```python
from build123d import *

# Parameters (mm, degrees)
SKETCH1_R           = 4.5
SKETCH1_R_2         = 2
BOSS_EXTRUDE1_DEPTH = 4


with BuildPart() as part:
    # Sketch1 → Boss-Extrude1 (new body)
    with BuildSketch(Plane(origin=(0, 0, 0), x_dir=(1, 0, 0), z_dir=(0, 1, 0))):
        with BuildLine():
            Line((-270, 15), (270, 15))
            ThreePointArc((270, 15), (285, 0), (270, -15))
            Line((270, -15), (-270, -15))
            ThreePointArc((-270, -15), (-285, 0), (-270, 15))
        make_face()
        with Locations(Location((-270, 0, 0), (0, 0, 270))):
            Circle(SKETCH1_R, mode=Mode.SUBTRACT)
        with Locations(Location((270, 0, 0), (0, 0, 270))):
            Circle(SKETCH1_R, mode=Mode.SUBTRACT)
        with Locations(Location((-150, 0, 0), (0, 0, 270))):
            Circle(SKETCH1_R_2, mode=Mode.SUBTRACT)
        with Locations(Location((150, 0, 0), (0, 0, 270))):
            Circle(SKETCH1_R_2, mode=Mode.SUBTRACT)
        with Locations(Location((0, 0, 0), (0, 0, 270))):
            Circle(SKETCH1_R_2, mode=Mode.SUBTRACT)
        with Locations(Location((-250, 0, 0), (0, 0, 270))):
            Circle(SKETCH1_R_2, mode=Mode.SUBTRACT)
        with Locations(Location((-230, 0, 0), (0, 0, 270))):
            Circle(SKETCH1_R_2, mode=Mode.SUBTRACT)
        with Locations(Location((-20, 0, 0), (0, 0, 270))):
            Circle(SKETCH1_R_2, mode=Mode.SUBTRACT)
        with Locations(Location((230, 0, 0), (0, 0, 90))):
            Circle(SKETCH1_R_2, mode=Mode.SUBTRACT)
        with Locations(Location((250, 0, 0), (0, 0, 90))):
            Circle(SKETCH1_R_2, mode=Mode.SUBTRACT)
        with Locations(Location((20, 0, 0), (0, 0, 90))):
            Circle(SKETCH1_R_2, mode=Mode.SUBTRACT)
    extrude(amount=BOSS_EXTRUDE1_DEPTH)


solid = part.part
```
Geometry check sheet. Reference: the model listing, model coordinates, mm. Give positions to 0.01 mm unless a question says otherwise; leave off trailing zeros. Write item = value, one per line. Start each with the question number.
1) Scan lines: L1, parallel to Z at x = 150, y = 1.1; L2, parallel to X at y = 2.5, z = 3.5; L3, parallel to X at y = 2.8, z = -7. Record each from-to range of solid material in increasing order.
2) Draft check along X on faces 1 (the cylindrical face through (-285, 2, 0)), 2 (the cylindrical face through (265.61, 1.97, -0.98)), 3 (the flat face through (4, 0, 0)). Enter one of: released by +X, released by -X, zero draft, split by the parting line, or undercut.
3) Gauge pin test, flat ends, axial feed: pin 1 Ø1 at (y, z) = (1, 2) entering from -X; pin 2 Ø2.5 at (x, z) = (-230, 0) entering from -Y. Record the tip position at first contact, or that the pin passes through.
4) Section check A-A (y = 3.05). Count the separate pieces of the cut face and the enclosed holes in it, then the cut area to 3 significant figures.
Geometry check:
q1.L1 = -15 to -2, 2 to 15
q1.L2 = -284.59 to -272.83, -267.17 to 267.17, 272.83 to 284.59
q1.L3 = -283.27 to 283.27
q2.face_1 = released by -X
q2.face_2 = undercut
q2.face_3 = zero draft
q3.pin_1 = -284.92
q3.pin_2 = through
q4.separate_pieces = 1
q4.enclosed_holes = 11
q4.area = 16,700 mm2
